The figure shows three views and two pictorial views of one solid part (mm, origin at its lowest corner). Answer the questions. A direction names the side the tool comes from. Coordinates: 2 decimals unless noted, no trailing zeros. Write each loop counter-clockwise with the first axis right and the second up, starting at its lowest first coordinate (ties: lowest second). Pieces come first, ordered by that corner, then holes. Notation, with made-up numbers: (54, 69) - (92, 69) arc R30 cw to (92, 102) - close; hole circle Ø8 at (53.5, -10.5). An arc over 180 degrees is marked (long way). Use a Markdown table: item, result. Add a question column.
(1) For a pull along Z with two mould halves and no side action, classify the marked faces 4, 5, 6 and 7 as released by +Z, released by -Z, zero draft, split by the parting line, or undercut.
(2) The part is cut by section A-A, the plane x = 269. Give the vertices of the cut face in (y, z) (1 decimal), then the cut area to 3 significant figures.
(3) Find the intervals of material crossed by line 1 (Z direction, x = 324, y = 2); line 2 (Z direction, x = 267, y = 22.5) (1 decimal); line 3 (X direction, y = 127, z = 67), in increasing order. Write a range as from..to.
(4) The part is cut by section C-C, the plane y = 40.5. Give the vertices of the cut face in (x, z) (1 decimal), then the cut area to 3 significant figures.
(5) The part is cut by section B-B, the plane x = 25.5. Give the vertices of the cut face in (y, z) (1 decimal).
(6) Given pin 1 Ø5 at (y, z) = (7, 65) entering from -X; pin 2 Ø8 at (x, z) = (36, 97) entering from +Y (1 decimal); pin 3 Ø6 at (x, y) = (154.5, 97.5) entering from +Z; pin 4 Ø6 at (x, y) = (162, 117.5) entering from -Z, each flat-ended and moving along its own axis, determine where each tip first touches the part or whether it passes through.
(7) A tool of negligible diameter and unlimited length cuts with its end or side. For the marked faces 1, 2 and 3, from which of +Z, -Z, +X, -X, +Y, -Y can it reach the whole face along a straight path? Write none if from no direction.
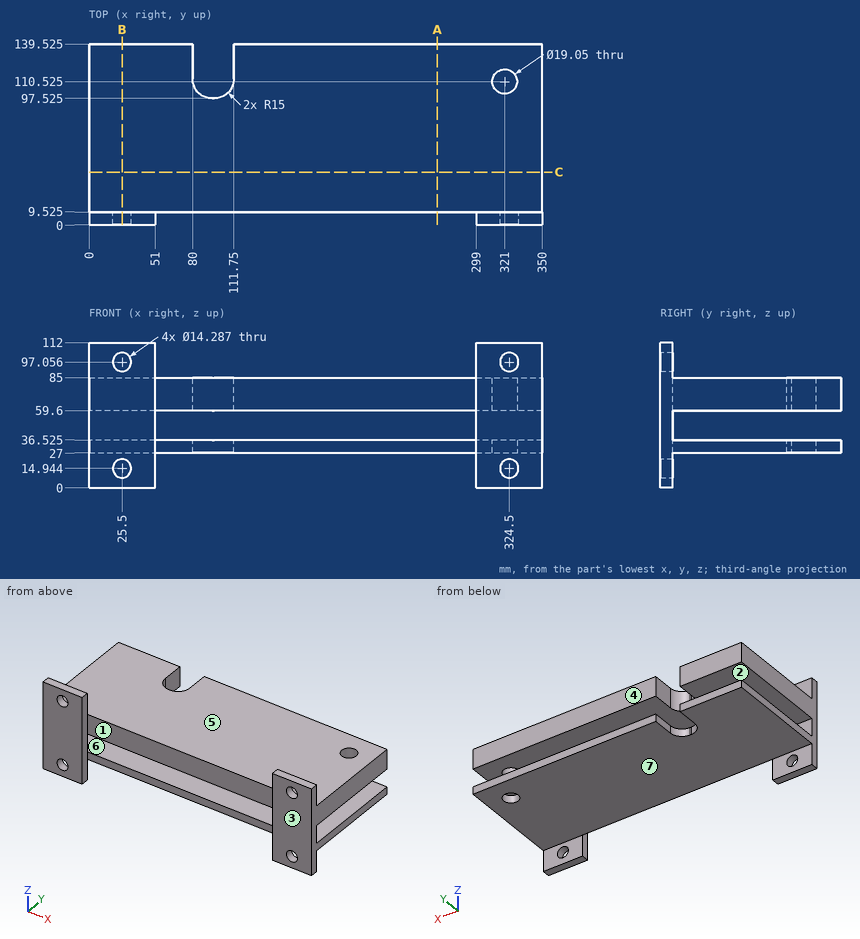
Model answer:
| question | item | result |
|---|---|---|
| 1 | face 4 | zero draft |
| 1 | face 5 | released by +Z |
| 1 | face 6 | undercut |
| 1 | face 7 | released by -Z |
| 2 | outline | (9.5, 27) - (139.5, 27) - (139.5, 36.5) - (9.5, 36.5) - close; (9.5, 59.6) - (139.5, 59.6) - (139.5, 85) - (9.5, 85) - close |
| 2 | area | 4,540 mm^2 |
| 3 | line 1 | 0..7.82, 22.07..89.93, 104.18..112 |
| 3 | line 2 | 27..36.5, 59.6..85 |
| 3 | line 3 | 0..80, 111.75..350 |
| 4 | outline | (0, 27) - (350, 27) - (350, 36.5) - (0, 36.5) - close; (0, 59.6) - (350, 59.6) - (350, 85) - (0, 85) - close |
| 4 | area | 12,200 mm^2 |
| 5 | outline | (0, 0) - (9.5, 0) - (9.5, 7.8) - (0, 7.8) - close; (0, 22.1) - (9.5, 22.1) - (9.5, 27) - (139.5, 27) - (139.5, 36.5) - (9.5, 36.5) - (9.5, 59.6) - (139.5, 59.6) - (139.5, 85) - (9.5, 85) - (9.5, 89.9) - (0, 89.9) - close; (0, 104.2) - (9.5, 104.2) - (9.5, 112) - (0, 112) - close |
| 6 | pin 1 | x = 0 |
| 6 | pin 2 | y = 9.5 |
| 6 | pin 3 | z = 85 |
| 6 | pin 4 | z = 27 |
| 7 | face 1 | +Z, -Z, -Y |
| 7 | face 2 | +X, -X, +Y |
| 7 | face 3 | +Z, -Z, +X, -X, -Y |
